Design review of the part built by this model. Coordinates are the model's own, in mm. Face numbers are marked on the shaded views. Give positions to 0.01 mm unless a question says otherwise; leave off trailing zeros. Loops run counter-clockwise (first coordinate to the right, second up) from the corner with the lowest first, then second, coordinate; pieces in that order, holes last. Notation, with made-up numbers: (2, -34) -> (44, -34) arc R22 cw to (44, -6) -> close; hole circle Ø4 at (26.5, -24). An arc over 180 degrees is marked (long way). Use a Markdown table: item, result. Add a question column.
1. To check wall thickness, follow line 1 (Z direction, x = 0, y = 96); line 2 (Y direction, x = 41, z = 7). State the ranges of each line that lie inside material, in increasing order.
2. Add section C-C (y = 66.5). State the section outline as (x, z) points.
3. For pin 1 Ø10 at (y, z) = (106.5, 14) entering from +X; pin 2 Ø8 at (x, y) = (-4, 118) entering from +Z; pin 3 Ø1.5 at (x, y) = (2.5, 22.5) entering from -Z, all flat-tipped, find the tip position at first contact; note any pin that passes through.
4. Add section B-B (z = 0). State the section outline as (x, y) points, and give its area (3 significant figures).
5. Draft analysis for pull direction Y (two halves, no side actions). For the marked faces 1 and 2, state which applies: pulls with the +Y half, pulls with the -Y half, needs draft (parallel to the pull), parting line crosses it, or undercut.
6. Add section A-A (x = 0). State the section outline as (y, z) points, and give its area (3 significant figures).
```python
from build123d import *

# Parameters (mm, degrees)
SCHIZZO1_R                   = 40
SCHIZZO1_R_2                 = 39
ESTRUSIONE_SOTTILE1_DEPTH    = 150
ESTRUSIONE_ESTRUSIONE1_START = -1
SCHIZZO2_R                   = 46
SCHIZZO2_R_2                 = 40
ESTRUSIONE_ESTRUSIONE1_DEPTH = 1
SCHIZZO3_R                   = 46
SCHIZZO3_R_2                 = 40
ESTRUSIONE_ESTRUSIONE2_DEPTH = 1


with BuildPart() as part:
    # Schizzo1 → Estrusione-Sottile1 (new body)
    with BuildSketch(Plane(origin=(0, 0, 0), x_dir=(1, 0, 0), z_dir=(0, 1, 0))):
        Circle(SCHIZZO1_R)
        Circle(SCHIZZO1_R_2, mode=Mode.SUBTRACT)
    extrude(amount=ESTRUSIONE_SOTTILE1_DEPTH)

    # Schizzo2 → Estrusione-Estrusione1 (add)
    with BuildSketch(Plane(origin=(0, 150, 0), x_dir=(1, 0, 0), z_dir=(0, 1, 0)).offset(ESTRUSIONE_ESTRUSIONE1_START)):
        with Locations(Location((0, 0, 0), (0, 0, 270))):
            Circle(SCHIZZO2_R)
        with Locations(Location((0, 0, 0), (0, 0, 270))):
            Circle(SCHIZZO2_R_2, mode=Mode.SUBTRACT)
    extrude(amount=ESTRUSIONE_ESTRUSIONE1_DEPTH)

    # Schizzo3 → Estrusione-Estrusione2 (add)
    with BuildSketch(Plane.XZ):
        with Locations(Location((0, 0, 0), (0, 0, 90))):
            Circle(SCHIZZO3_R)
        with Locations(Location((0, 0, 0), (0, 0, 270))):
            Circle(SCHIZZO3_R_2, mode=Mode.SUBTRACT)
    extrude(amount=-ESTRUSIONE_ESTRUSIONE2_DEPTH)


solid = part.part
```
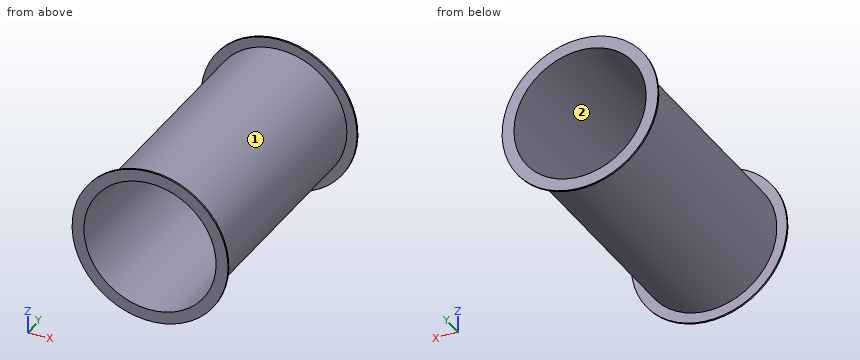
Taken from the geometry:
| question | item | result |
|---|---|---|
| 1 | line 1 | z = -40 to -39, 39 to 40 |
| 1 | line 2 | y = 0 to 1, 149 to 150 |
| 2 | outline | circle Ø80 at (0, 0); hole circle Ø78 at (0, 0) |
| 3 | pin 1 | stops at x = 38.97 |
| 3 | pin 2 | stops at z = 40 |
| 3 | pin 3 | stops at z = -39.96 |
| 4 | outline | (-46, 0) -> (-39, 0) -> (-39, 150) -> (-46, 150) -> (-46, 149) -> (-40, 149) -> (-40, 1) -> (-46, 1) -> close; (39, 0) -> (46, 0) -> (46, 1) -> (40, 1) -> (40, 149) -> (46, 149) -> (46, 150) -> (39, 150) -> close |
| 4 | area | 324 mm^2 |
| 5 | face 1 | undercut |
| 5 | face 2 | needs draft |
| 6 | outline | (0, -46) -> (1, -46) -> (1, -40) -> (149, -40) -> (149, -46) -> (150, -46) -> (150, -39) -> (0, -39) -> close; (0, 39) -> (150, 39) -> (150, 46) -> (149, 46) -> (149, 40) -> (1, 40) -> (1, 46) -> (0, 46) -> close |
| 6 | area | 324 mm^2 |
